```python
from build123d import *

# Parameters (mm, degrees)
SKETCH1_R           = 14.5
SKETCH1_R_2         = 1.5
BOSS_EXTRUDE1_DEPTH = 4
BOSS_EXTRUDE2_DEPTH = 25
CHAMFER1_SIZE       = 5


with BuildPart() as part:
    # Sketch1 → Boss-Extrude1 (new body)
    with BuildSketch(Plane.XY):
        with Locations((43.483141232, -69.989052064)):
            Circle(SKETCH1_R)
        with Locations((43.483141232, -58.489052064)):
            Circle(SKETCH1_R_2, mode=Mode.SUBTRACT)
        with Locations((54.983141232, -69.989052064)):
            Circle(SKETCH1_R_2, mode=Mode.SUBTRACT)
        with Locations((31.983141232, -69.989052064)):
            Circle(SKETCH1_R_2, mode=Mode.SUBTRACT)
        with Locations((43.483141232, -81.489052064)):
            Circle(SKETCH1_R_2, mode=Mode.SUBTRACT)
    extrude(amount=BOSS_EXTRUDE1_DEPTH)

    # Sketch2 → Boss-Extrude2 (add)
    with BuildSketch(Plane.XY.offset(4)):
        Polygon((47.524593117, -69.989052064), (45.503867174, -66.489052064), (41.46241529, -66.489052064), (39.441689348, -69.989052064), (41.46241529, -73.489052064), (45.503867174, -73.489052064), align=None)
    extrude(amount=BOSS_EXTRUDE2_DEPTH)

    # Chamfer1
    chamfer1_edges = [part.edges().sort_by_distance(p)[0] for p in [
        (46.514230145, -71.739052064, 4),
        (46.514230145, -68.239052064, 4),
        (43.483141232, -66.489052064, 4),
        (40.452052319, -68.239052064, 4),
        (40.452052319, -71.739052064, 4),
        (43.483141232, -73.489052064, 4),
    ]]
    chamfer(chamfer1_edges, length=CHAMFER1_SIZE)


solid = part.part
```
The listing builds one solid part. Answer for the finished solid, in the listing's coordinates (mm). A direction names the side the tool comes from. Round coordinates to 2 decimals unless told otherwise and drop trailing zeros. Write each loop counter-clockwise with the first axis right and the second up, starting at its lowest first coordinate (ties: lowest second). Pieces come first, ordered by that corner, then holes. Notation, with made-up numbers: (62.5, 17) -> (68.5, 17) arc R15 cw to (68.5, 37) -> close; hole circle Ø2 at (8.5, 49). An arc over 180 degrees is marked (long way). Write item = value, one per line.
1) Section A-A on y = -80.5 is taken. Write down the section's boundary in (x, z), plus the area to 3 significant figures.
Check values:
outline = (33.49, 0) -> (42.36, 0) -> (42.36, 4) -> (33.49, 4) -> close; (44.61, 0) -> (53.47, 0) -> (53.47, 4) -> (44.61, 4) -> close
area = 70.9 mm²
2) Which of the six approach directions +Z, -Z, +X, -X, +Y, -Y give full straight-line access (tool end or side, diameter ignored) to faces 4 (the flat face through (44, -66.489, 19)), 5 (the flat face through (43, -73.489, 19)), 6 (the flat face through (40.438, -71.715, 18.86)), 7 (the flat face through (46.5, -71.76, 18.86))?
Check values:
face_4 = +Z, +X, -X, +Y
face_5 = +Z, +X, -X, -Y
face_6 = +Z, -X, -Y
face_7 = +Z, +X, -Y
3) Section B-B on z = 16.5 is taken. Write down the section's boundary in (x, y).
Check values:
outline = (39.44, -69.99) -> (41.46, -73.49) -> (45.5, -73.49) -> (47.52, -69.99) -> (45.5, -66.49) -> (41.46, -66.49) -> close
4) For a pull along X with two mould halves and no side action, classify faces 1 (the cylindrical face through (42.378, -80.475, 1.972)), 2 (the flat face through (37.8, -73.19, 5.98)), 3 (the flat face through (49.164, -66.788, 5.979)) as released by +X, released by -X, zero draft, split by the parting line, or undercut.
Check values:
face_1 = undercut
face_2 = released by -X
face_3 = released by +X
5) Section D-D on y = -63.25 is taken. Write down the section's boundary in (x, z), plus the area to 3 significant figures.
Check values:
outline = (30.64, 0) -> (56.32, 0) -> (56.32, 4) -> (49.41, 4) -> (47.37, 5.76) -> (39.59, 5.76) -> (37.56, 4) -> (30.64, 4) -> close
area = 120 mm²
6) Given pin 1 (2 mm diameter, centred on x = 44, z = 14.5, fed in from +Y); pin 2 (1 mm diameter, centred on x = 37.5, z = 20, fed in from +Y); pin 3 (2 mm diameter, centred on x = 42.5, z = 22.5, fed in from -Y); pin 4 (1.5 mm diameter, centred on y = -58.5, z = 4, fed in from +X), each flat-ended and moving along its own axis, determine where each tip first touches the part or whether it passes through.
Check values:
pin_1 = -66.49
pin_2 = through
pin_3 = -73.49
pin_4 = 53.23
7) Straight lines are drawn through the part: line 1 along Z through (x, y) = (37.25, -82.75); line 2 along Z through (x, y) = (43, -74); line 3 along Y through (x, z) = (45, 8). For each, find the intervals that lie inside material, in ascending order. Write a range as [from, to].
Check values:
line_1 = [0, 4]
line_2 = [0, 8.49]
line_3 = [-74.49, -65.49]
8) Section C-C on y = -75 is taken. Write down the section's boundary in (x, z).
Check values:
outline = (29.88, 0) -> (57.09, 0) -> (57.09, 4) -> (50.41, 4) -> (46.38, 7.49) -> (40.59, 7.49) -> (36.56, 4) -> (29.88, 4) -> close
